Part model, mm, in its own coordinate system. Give positions to 0.01 mm unless a question says otherwise; leave off trailing zeros. Write each loop counter-clockwise with the first axis right and the second up, starting at its lowest first coordinate (ties: lowest second). Pieces come first, ordered by that corner, then holes. Notation, with made-up numbers: M 82.5,6.5 L 134.5,6.5 A5 ccw 134.5,14.5 Z; hole C -9.75,82.25 d2. An arc over 180 degrees is marked long. Use CSV: the item, a comma, the result in double quotes. Start each with the question number.
Item 1: Cut at A-A (y = -20). List the corners of the cut face in (x, z), then the cut area to 3 significant figures.
Item 2: Cut at B-B (x = 12.5). List the corners of the cut face in (y, z), then the cut area to 3 significant figures.
Item 3: Cut at C-C (z = 1). List the corners of the cut face in (x, y).
Item 4: Drill centre lines: line 1 (Y direction, x = 255.5, z = 2.25); line 2 (Y direction, x = 12.5, z = 2.5); line 3 (X direction, y = -178, z = -3). Where is each one in solid material? Low to high. Write a range as [from, to].
Item 5: Pin check, flat tips, straight feed: pin 1 (2.5 mm diameter, centred on x = 173.5, y = -178, fed in from +Z); pin 2 (5 mm diameter, centred on x = 147.5, z = 0.5, fed in from +Y). Stop position of each tip, or through.
Item 6: Cut at D-D (y = -43). List the corners of the cut face in (x, z), then the cut area to 3 significant figures.
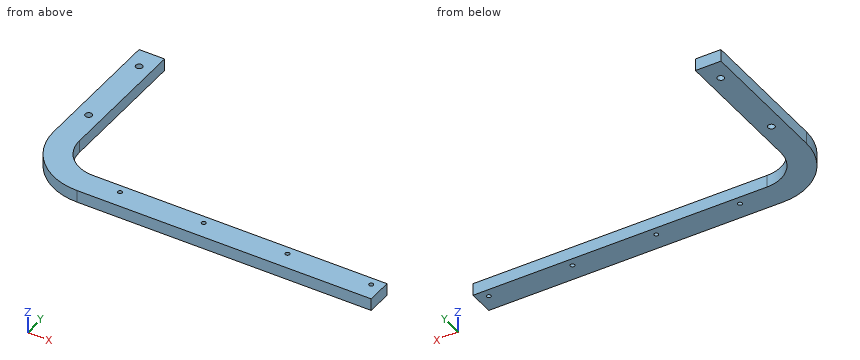
from build123d import *

# Parameters (mm, degrees)
BOSS_EXTRUDE1_DEPTH  = 6
M6_CLEARANCE_HOLE1_D = 6.6
M5_TAPPED_HOLE1_D    = 4.2
LPATTERN1_COUNT      = 4
LPATTERN1_PITCH      = 82


with BuildPart() as part:
    # Sketch1 → Boss-Extrude1 (new body, symmetric)
    with BuildSketch(Plane.XY):
        with BuildLine():
            Line((0, 0), (0, -135))
            ThreePointArc((0, -135), (17.573593129, -177.426406871), (60, -195))
            Line((60, -195), (348, -195))
            Line((348, -195), (348, -170))
            Line((348, -170), (60, -170))
            ThreePointArc((60, -170), (35.251262658, -159.748737342), (25, -135))
            Line((25, -135), (25, 0))
            Line((25, 0), (0, 0))
        make_face()
    extrude(amount=BOSS_EXTRUDE1_DEPTH, both=True)

    # M6 Clearance Hole1 (through all)
    with Locations(Plane.XY.offset(6)):
        with Locations((12.5, -20), (12.5, -100)):
            Hole(M6_CLEARANCE_HOLE1_D / 2)

    # M5 Tapped Hole1 (through all)
    with Locations(Plane.XY.offset(6)):
        with Locations((337.5, -178)):
            m5_tapped_hole1 = Hole(M5_TAPPED_HOLE1_D / 2)

    # LPattern1: M5 Tapped Hole1 ×4
    with Locations(*[(-i * LPATTERN1_PITCH, 0, 0) for i in range(1, LPATTERN1_COUNT)]):
        add(m5_tapped_hole1, mode=Mode.SUBTRACT)


solid = part.part
Worked answers:
1,outline,"M 0,-6 L 9.2,-6 L 9.2,6 L 0,6 Z; M 15.8,-6 L 25,-6 L 25,6 L 15.8,6 Z"
1,area,"221 mm^2"
2,outline,"M -171.66,-6 L -103.3,-6 L -103.3,6 L -171.66,6 Z; M -96.7,-6 L -23.3,-6 L -23.3,6 L -96.7,6 Z; M -16.7,-6 L 0,-6 L 0,6 L -16.7,6 Z"
2,area,"1,900 mm^2"
3,outline,"M 0,-135 A60 ccw 60,-195 L 348,-195 L 348,-170 L 60,-170 A35 cw 25,-135 L 25,0 L 0,0 Z; hole C 12.5,-100 d6.6; hole C 12.5,-20 d6.6; hole C 91.5,-178 d4.2; hole C 173.5,-178 d4.2; hole C 255.5,-178 d4.2; hole C 337.5,-178 d4.2"
4,line 1,"y = [-195, -180.1], [-175.9, -170]"
4,line 2,"y = [-171.66, -103.3], [-96.7, -23.3], [-16.7, 0]"
4,line 3,"x = [18.16, 89.4], [93.6, 171.4], [175.6, 253.4], [257.6, 335.4], [339.6, 348]"
5,pin 1,"passes through"
5,pin 2,"stops at y = -170"
6,outline,"M 0,-6 L 25,-6 L 25,6 L 0,6 Z"
6,area,"300 mm^2"
